Could you check a few things on this model? Use its own coordinates, in mm. Face numbers are marked on the shaded views. Coordinates: 2 decimals unless noted, no trailing zeros. Write each loop counter-clockwise with the first axis right and the second up, starting at its lowest first coordinate (ties: lowest second). Pieces come first, ordered by that corner, then holes. Notation, with made-up numbers: M -7.5,23 L 41.5,23 A27 ccw 41.5,44 Z; hole C -36,26 d3. An arc over 180 degrees is marked long. Answer as CSV lines item,"result". Start each with the question number.
Item 1: We'd pull the mould along Y, two halves only. Please class the marked faces 1, 2 and 3: +Y half, -Y half, draft (parallel to the pull), parting line (faces both ways), or undercut.
Item 2: If I drill on line 1 along Y through (x, z) = (-9, 4.2); line 2 along X through (y, z) = (0.25, 0.55); line 3 along X through (y, z) = (0.75, 2.9), over which ranges is the centre line in solid material (lowest first)? Write a range as [from, to].
Item 3: Suppose I cut it at A-A, the plane y = 0. Write out the boundary of the cut face in (x, z).
Item 4: I'm going to push a flat-ended pin straight in: P1, Ø5, axis at x = 9, y = 0, coming from the +Z side. Where does the tip first touch, or does it pass through?
Item 5: Suppose I cut it at C-C, the plane z = 4.75. Write out the boundary of the cut face in (x, y), and give its area (3 significant figures).
Item 6: Suppose I cut it at B-B, the plane x = -9. Write out the boundary of the cut face in (y, z).
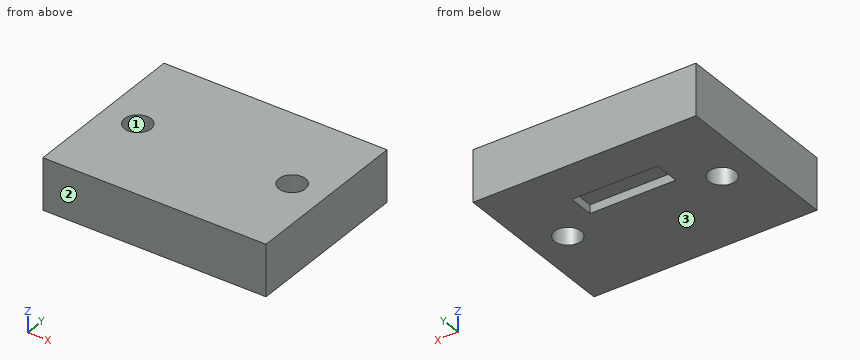
```python
from build123d import *

# Parameters (mm, degrees)
SKETCH1_W           = 26
SKETCH1_H           = 20
SKETCH1_R           = 1.55
BOSS_EXTRUDE1_DEPTH = 6
SKETCH4_W           = 10
SKETCH4_H           = 2
CUT_EXTRUDE3_DEPTH  = 1
CHAMFER1_SIZE       = 1


with BuildPart() as part:
    # Sketch1 → Boss-Extrude1 (new body)
    with BuildSketch(Plane.XY):
        Rectangle(SKETCH1_W, SKETCH1_H)
        with Locations((9, 0)):
            Circle(SKETCH1_R, mode=Mode.SUBTRACT)
        with Locations((-9, 0)):
            Circle(SKETCH1_R, mode=Mode.SUBTRACT)
    extrude(amount=BOSS_EXTRUDE1_DEPTH)

    # Sketch4 → Cut-Extrude3 (cut)
    with BuildSketch(Plane(origin=(0, 0, 0), x_dir=(-1, 0, 0), z_dir=(0, 0, -1))):
        with Locations((0, 3)):
            Rectangle(SKETCH4_W, SKETCH4_H)
    extrude(amount=-CUT_EXTRUDE3_DEPTH, mode=Mode.SUBTRACT)

    # Chamfer1
    chamfer1_edges = [part.edges().sort_by_distance(p)[0] for p in [
        (0, 4, 0),
    ]]
    chamfer(chamfer1_edges, length=CHAMFER1_SIZE - 0.0001)  # a hair under: the kernel refuses the full size


solid = part.part
```
Ans:
1,face 1,"undercut"
1,face 2,"-Y half"
1,face 3,"draft"
2,line 1,"y = [-10, -1.55], [1.55, 10]"
2,line 2,"x = [-13, -10.53], [-7.47, 7.47], [10.53, 13]"
2,line 3,"x = [-13, -10.36], [-7.64, 7.64], [10.36, 13]"
3,outline,"M -13,0 L -10.55,0 L -10.55,6 L -13,6 Z; M -7.45,0 L 7.45,0 L 7.45,6 L -7.45,6 Z; M 10.55,0 L 13,0 L 13,6 L 10.55,6 Z"
4,P1,"stops at z = 6"
5,outline,"M -13,-10 L 13,-10 L 13,10 L -13,10 Z; hole C -9,0 d3.1; hole C 9,0 d3.1"
5,area,"505 mm^2"
6,outline,"M -10,0 L -1.55,0 L -1.55,6 L -10,6 Z; M 1.55,0 L 10,0 L 10,6 L 1.55,6 Z"
